Could you check a few things on this model? Use its own coordinates, in mm. Round coordinates to 2 decimals unless told otherwise and drop trailing zeros. Order: outer loops, then holes, each group sorted by start corner. A loop starts at its lowest first (then second) coordinate and runs counter-clockwise, first axis right, second up. Notation, with made-up numbers: (-8.5, 80) -> (28.5, 80) arc R20 ccw to (28.5, 96) -> close; hole circle Ø11 at (-39, 86.25). An arc over 180 degrees is marked (long way). One line per question, with ' | ' between items.
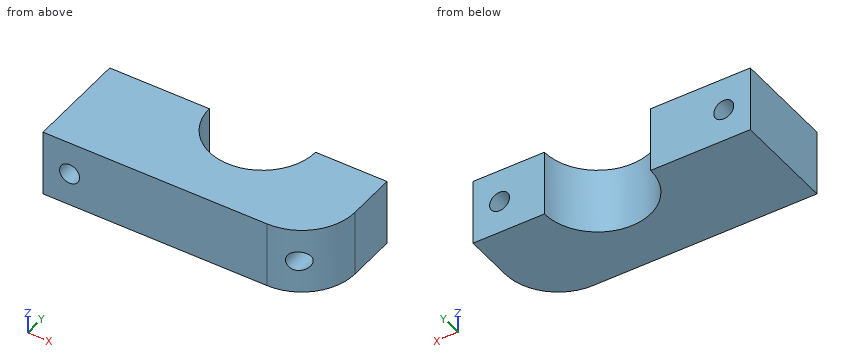
```python
from build123d import *

# Parameters (mm, degrees)
BOSS_EXTRUDE1_DEPTH = 10
SKETCH2_R           = 1.5
CUT_EXTRUDE1_DEPTH  = 46.609456256


with BuildPart() as part:
    # Sketch1 → Boss-Extrude1 (new body)
    with BuildSketch(Plane.XY):
        with BuildLine():
            Line((0, 0), (-10.75, 0))
            ThreePointArc((-10.75, 0), (-18.75, -8), (-26.75, 0))
            Line((-26.75, 0), (-41.75, 0))
            Line((-41.75, 0), (-41.75, -15.4))
            Line((-41.75, -15.4), (-8, -15.4))
            ThreePointArc((-8, -15.4), (-2.343145751, -13.056854249), (0, -7.4))
            Line((0, -7.4), (0, 0))
        make_face()
    extrude(amount=BOSS_EXTRUDE1_DEPTH)

    # Sketch2 → Cut-Extrude1 (cut, through all)
    with BuildSketch(Plane.XZ.offset(15.4)):
        with Locations(Location((-37.75, 5, 0), (0, 0, 270))):
            Circle(SKETCH2_R)
        with Locations(Location((-4, 5, 0), (0, 0, 270))):
            Circle(SKETCH2_R)
    extrude(amount=-CUT_EXTRUDE1_DEPTH, mode=Mode.SUBTRACT)


solid = part.part
```
1. I want a section at C-C on z = 2.5. List the corners of the cut face in (x, y) for me, and give its area (3 significant figures).
From the geometry:
outline: (-41.75, -15.4) -> (-8, -15.4) arc R8 ccw to (0, -7.4) -> (0, 0) -> (-10.75, 0) arc R8 cw to (-26.75, 0) -> (-41.75, 0) -> close | area: 529 mm²
2. I want a section at D-D on y = -13. List the corners of the cut face in (x, z) for me.
From the geometry:
outline: (-41.75, 0) -> (-2.29, 0) -> (-2.29, 10) -> (-41.75, 10) -> close; hole circle Ø3 at (-37.75, 5); hole circle Ø3 at (-4, 5)
3. I'm going to push flat-ended pins straight in: pin 1 (5 mm diameter, centred on x = -4, z = 5, fed in from -Y); pin 2 (2 mm diameter, centred on x = -17.5, z = 4, fed in from +Y); pin 3 (2 mm diameter, centred on y = -9, z = 8, fed in from +X). Where does each tip first touch, or does it pass through?
From the geometry:
pin 1: stops at y = -15.26 | pin 2: stops at y = -7.68 | pin 3: stops at x = -0.02
4. I need wall thicknesses on probe 1 along X at (y, z) = (-13.5, 5); probe 2 along X at (y, z) = (-6.25, 5); probe 3 along Z at (x, y) = (-4, -10). Which ranges of each line are inside material? Lowest first, please.
From the geometry:
probe 1: x = -41.75 to -39.25, -36.25 to -5.5 | probe 2: x = -41.75 to -39.25, -36.25 to -23.74, -13.76 to -5.5, -2.5 to 0 | probe 3: z = 0 to 3.5, 6.5 to 10
5. I want a section at B-B on x = -37.75. List the corners of the cut face in (y, z) for me, and give its area (3 significant figures).
From the geometry:
outline: (-15.4, 0) -> (0, 0) -> (0, 3.5) -> (-15.4, 3.5) -> close; (-15.4, 6.5) -> (0, 6.5) -> (0, 10) -> (-15.4, 10) -> close | area: 108 mm²
6. I want a section at A-A on y = -3.25. List the corners of the cut face in (x, z) for me, and give its area (3 significant figures).
From the geometry:
outline: (-41.75, 0) -> (-26.06, 0) -> (-26.06, 10) -> (-41.75, 10) -> close; (-11.44, 0) -> (0, 0) -> (0, 10) -> (-11.44, 10) -> close; hole circle Ø3 at (-37.75, 5); hole circle Ø3 at (-4, 5) | area: 257 mm²
